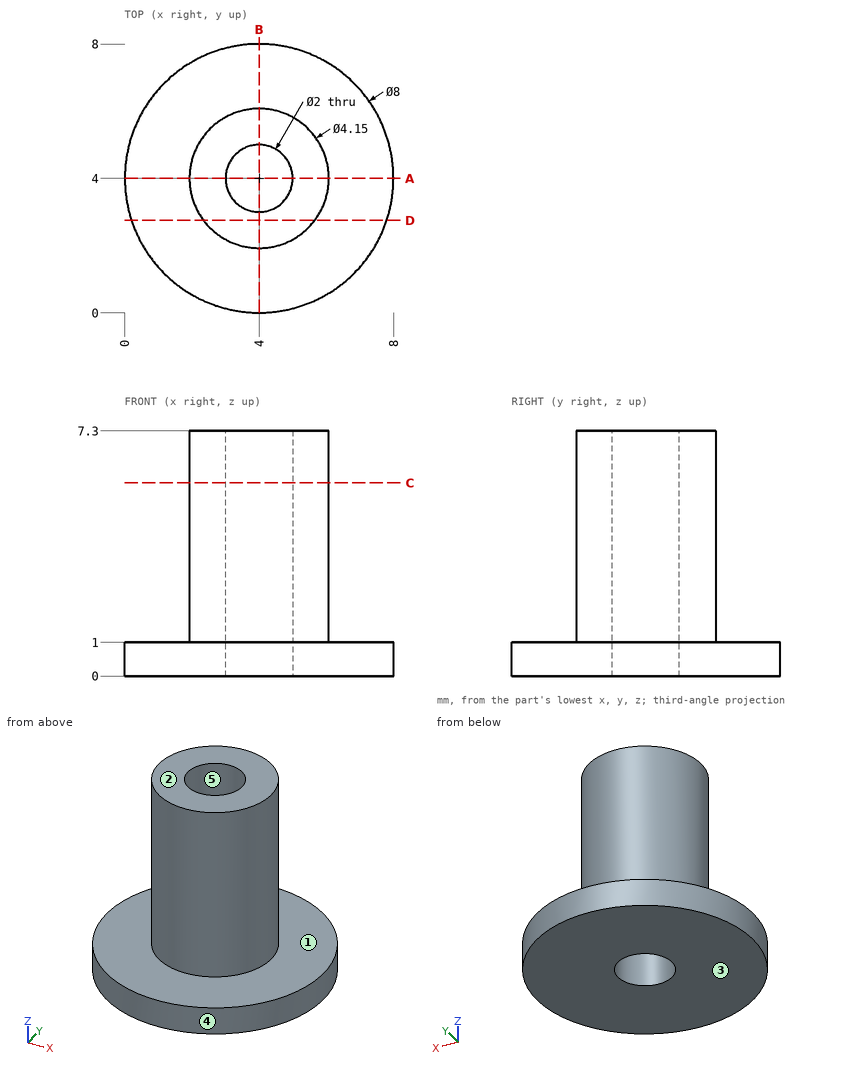
Part print with two shaded views. Sizes in mm from the minimum x, y, z corner. A direction names the side the tool comes from. Give positions to 0.01 mm unless a question says otherwise; leave off trailing zeros. Write each loop counter-clockwise with the first axis right and the second up, starting at its lowest first coordinate (ties: lowest second). Pieces come first, ordered by that corner, then holes.
1) Cut at D-D on y = 2.75. Write the cut outline in (x, z), then the cut area to 3 significant figures.
Resolved:
outline: (0.2, 0) - (7.8, 0) - (7.8, 1) - (5.66, 1) - (5.66, 7.3) - (2.34, 7.3) - (2.34, 1) - (0.2, 1) - close
area: 28.5 mm2
2) Which spindle directions (+Z, -Z, +X, -X, +Y, -Y) get a long thin tool onto all of the face, cutting with end or side? Do the marked faces 1 and 2. Say none if no direction does.
Resolved:
face 1: +Z
face 2: +Z, +X, -X, +Y, -Y
3) Cut at A-A on y = 4. Write the cut outline in (x, z) (3 decimals), then the cut area to 3 significant figures.
Resolved:
outline: (0, 0) - (3, 0) - (3, 7.3) - (1.925, 7.3) - (1.925, 1) - (0, 1) - close; (5, 0) - (8, 0) - (8, 1) - (6.075, 1) - (6.075, 7.3) - (5, 7.3) - close
area: 19.5 mm2
4) Two-plate mould, pull along X, no slides. Class the marked faces 3, 4 and 5: released by +X, released by -X, zero draft, split by the parting line, or undercut.
Resolved:
face 3: zero draft
face 4: split by the parting line
face 5: undercut
5) Cut at C-C on z = 5.75. Write the cut outline in (x, y) (3 decimals), then the cut area to 3 significant figures.
Resolved:
outline: circle Ø4.15 at (4, 4); hole circle Ø2 at (4, 4)
area: 10.4 mm2
6) Pin check, flat tips, straight feed: pin 1 (3 mm diameter, centred on x = 3.5, z = 6.5, fed in from -Y) (3 decimals); pin 2 (2 mm diameter, centred on y = 2, z = 3.5, fed in from +X); pin 3 (3 mm diameter, centred on y = 4, z = 5.5, fed in from -X) (3 decimals). Stop position of each tip, or through.
Resolved:
pin 1: stops at y = 1.925
pin 2: stops at x = 5.82
pin 3: stops at x = 1.925
7) Probe L1, parallel to Y at x = 4, z = 2.25 (3 decimals); L2, parallel to Z at x = 3.75, y = 7.5; L3, parallel to X at y = 4.25, z = 1.75. List the from-to ranges inside material, lowest first.
Resolved:
L1: y = 1.925 to 3, 5 to 6.075
L2: z = 0 to 1
L3: x = 1.94 to 3.03, 4.97 to 6.06
